Check sheet for the modelled part. Datum: model origin and axes. Units: mm. A direction names the side the tool comes from. Give positions to 0.01 mm unless a question says otherwise; leave off trailing zeros. Order: outer loops, then holes, each group sorted by start corner. A loop starts at its lowest first (then second) coordinate and runs counter-clockwise, first axis right, second up.
```python
from build123d import *

# Parameters (mm, degrees)
F0_W     = 58
F0_H     = 23
F0_W_2   = 55
F0_H_2   = 20
F1_DEPTH = 150
F2_R     = 1
F3_R     = 1.5
F4_DEPTH = 15
F5_DEPTH = 15
F6_DEPTH = 15


with BuildPart() as f1:
    # F0 (on Front) → F1 (new body)
    with BuildSketch(Plane.XZ):
        Rectangle(F0_W, F0_H)
        Rectangle(F0_W_2, F0_H_2, mode=Mode.SUBTRACT)
    extrude(amount=F1_DEPTH)

    # F2
    f2_edges = [f1.edges().sort_by_distance(p)[0] for p in [
        (-29, -75, 11.5),
        (29, -75, 11.5),
        (-29, -75, -11.5),
        (29, -75, -11.5),
    ]]
    fillet(f2_edges, radius=F2_R)

    # F3 (on Top) → F4 (cut, symmetric)
    with BuildSketch(Plane.XY):
        with Locations((-19.25, -5)):
            Circle(F3_R)
    extrude(amount=F4_DEPTH, both=True, mode=Mode.SUBTRACT)

    # F3 (on Top) → F5 (cut, symmetric)
    with BuildSketch(Plane.XY):
        with Locations((19.25, -5)):
            Circle(F3_R)
    extrude(amount=F5_DEPTH, both=True, mode=Mode.SUBTRACT)

    # F3 (on Top) → F6 (cut, symmetric)
    with BuildSketch(Plane.XY):
        with Locations((19.25, -145)):
            Circle(F3_R)
        with Locations((-19.25, -145)):
            Circle(F3_R)
    extrude(amount=F6_DEPTH, both=True, mode=Mode.SUBTRACT)


solid = f1.part
```
(1) Sectioned sample at A-A (y = -5). Enter the section's corners in (x, z).
(2) Release check for a two-part mould opening along Y. For faces 3 (the face through (17.75, -4.93, 10.76)), 4 (the face through (-27.5, -74, 0)), 5 (the face through (-2.3, 0, -10.2)), 6 (the face through (17.75, -4.93, -10.74)) record: released by +Y, released by -Y, zero draft, split by the parting line, or undercut.
(3) Thickness scan on L1, parallel to X at y = -145, z = -10.7; L2, parallel to Y at x = 19.25, z = 10.8; L3, parallel to Z at x = 22, y = -118. Record the ranges inside material, lowest first.
(4) Tool access check on faces 1 (the face through (29, -74, 0)), 2 (the face through (0, -74, -10)). Record the directions out of +Z, -Z, +X, -X, +Y, -Y that give a thin tool (end or side, any length) a straight path to the whole face; none if there is none.
(5) Sectioned sample at C-C (z = 5.25). Enter the section's corners in (x, y).
(6) Sectioned sample at B-B (x = -19.25). Enter the section's corners in (y, z), plus the area to 3 significant figures.
(7) Sectioned sample at D-D (x = 8). Enter the section's corners in (y, z).
(8) Go/stop test with flat-tipped pins: P1, Ø3.5, axis at x = 19.25, y = -145, coming from the +Z side; P2, Ø1.8, axis at x = 19.25, y = -5, coming from the -Z side. Record where each tip stops, or that it passes through.
Values follow:
1. outline: (-29, -10.5) arc R1 ccw to (-28, -11.5) - (-20.75, -11.5) - (-20.75, -10) - (-27.5, -10) - (-27.5, 10) - (-20.75, 10) - (-20.75, 11.5) - (-28, 11.5) arc R1 ccw to (-29, 10.5) - close; (-17.75, -11.5) - (17.75, -11.5) - (17.75, -10) - (-17.75, -10) - close; (-17.75, 10) - (17.75, 10) - (17.75, 11.5) - (-17.75, 11.5) - close; (20.75, -11.5) - (28, -11.5) arc R1 ccw to (29, -10.5) - (29, 10.5) arc R1 ccw to (28, 11.5) - (20.75, 11.5) - (20.75, 10) - (27.5, 10) - (27.5, -10) - (20.75, -10) - close
2. face 3: undercut
2. face 4: zero draft
2. face 5: released by +Y
2. face 6: undercut
3. L1: x = -28.98 to -20.75, -17.75 to 17.75, 20.75 to 28.98
3. L2: y = -150 to -146.5, -143.5 to -6.5, -3.5 to 0
3. L3: z = -11.5 to -10, 10 to 11.5
4. face 1: +Z, -Z, +X, +Y, -Y
4. face 2: +Y, -Y
5. outline: (-29, -150) - (-27.5, -150) - (-27.5, 0) - (-29, 0) - close; (27.5, -150) - (29, -150) - (29, 0) - (27.5, 0) - close
6. outline: (-150, -11.5) - (-146.5, -11.5) - (-146.5, -10) - (-150, -10) - close; (-150, 10) - (-146.5, 10) - (-146.5, 11.5) - (-150, 11.5) - close; (-143.5, -11.5) - (-6.5, -11.5) - (-6.5, -10) - (-143.5, -10) - close; (-143.5, 10) - (-6.5, 10) - (-6.5, 11.5) - (-143.5, 11.5) - close; (-3.5, -11.5) - (0, -11.5) - (0, -10) - (-3.5, -10) - close; (-3.5, 10) - (0, 10) - (0, 11.5) - (-3.5, 11.5) - close
6. area: 432 mm2
7. outline: (-150, -11.5) - (0, -11.5) - (0, -10) - (-150, -10) - close; (-150, 10) - (0, 10) - (0, 11.5) - (-150, 11.5) - close
8. P1: stops at z = 11.5
8. P2: passes through
